```python
from build123d import *

# Parameters (mm, degrees)
SKETCH1_R           = 6.35
BOSS_EXTRUDE1_DEPTH = 22.86
SKETCH2_R           = 3.048
CUT_EXTRUDE1_DEPTH  = 8.636
SKETCH3_R           = 3.2385
CUT_EXTRUDE2_DEPTH  = 10.16


with BuildPart() as part:
    # Sketch1 → Boss-Extrude1 (new body)
    with BuildSketch(Plane(origin=(0, 0, 0), x_dir=(1, 0, 0), z_dir=(0, 1, 0))):
        Circle(SKETCH1_R)
    extrude(amount=BOSS_EXTRUDE1_DEPTH)

    # Sketch2 → Cut-Extrude1 (cut)
    with BuildSketch(Plane.XZ):
        Circle(SKETCH2_R)
    extrude(amount=-CUT_EXTRUDE1_DEPTH, mode=Mode.SUBTRACT)

    # Sketch3 → Cut-Extrude2 (cut)
    with BuildSketch(Plane(origin=(0, 22.86, 0), x_dir=(1, 0, 0), z_dir=(0, 1, 0))):
        Circle(SKETCH3_R)
    extrude(amount=-CUT_EXTRUDE2_DEPTH, mode=Mode.SUBTRACT)


solid = part.part
```
Design review of the part built by this model. Coordinates are the model's own, in mm. A direction names the side the tool comes from. Coordinates: 2 decimals unless noted, no trailing zeros. Order: outer loops, then holes, each group sorted by start corner. A loop starts at its lowest first (then second) coordinate and runs counter-clockwise, first axis right, second up. Notation, with made-up numbers: M 3,73 L 13,73 A29 cw 13,106 Z; hole C 71.25,23.5 d6. An arc over 180 degrees is marked long. Answer as a JSON object with one key per item and string values. Group by question number.
1) Add section A-A, the plane x = 0. Write out the cut boundary in (y, z).
2) Add section B-B, the plane z = 0. Write out the cut boundary in (x, y), then the cut area to 3 significant figures.
3) Wall thickness on L1, parallel to X at y = 19.5, z = 0; L2, parallel to Z at x = 0, y = 3.25: over which ranges is each line inside the solid? List them lowest first.
4) Add section C-C, the plane y = 7.5. Write out the cut boundary in (x, z), then the cut area to 3 significant figures.
5) Add section D-D, the plane y = 17. Write out the cut boundary in (x, z), then the cut area to 3 significant figures.
6) For pin 1 (4 mm diameter, centred on x = 0.5, y = 19.5, fed in from -Z); pin 2 (1.9 mm diameter, centred on x = 0, z = -1.5, fed in from +Y); pin 3 (3 mm diameter, centred on x = -3.5, y = 19, fed in from +Z); pin 4 (3 mm diameter, centred on y = 17.5, z = -3, fed in from -X), all flat-tipped, find the tip position at first contact; note any pin that passes through.
7) Tool access review of faces 1 (the flat face through (0, 12.7, 0)), 2 (the flat face through (0, 8.636, 0)), 3 (the flat face through (3, 0, -2)): name each direction out of +Z, -Z, +X, -X, +Y, -Y from which nothing blocks a thin tool from reaching the whole face with its end or side.
8) Mouldability with a two-part tool opening along X and no side actions: class faces 4 (the cylindrical face through (-1.38, 11.27, 6.2)), 5 (the cylindrical face through (-0.4, 4.26, 3.02)), 6 (the flat face through (-3, 22.86, -2)) as pulls with the +X half, pulls with the -X half, needs draft (parallel to the pull), parting line crosses it, or undercut.
Computed values:
{
 "1": {"outline": "M 0,-6.35 L 22.86,-6.35 L 22.86,-3.24 L 12.7,-3.24 L 12.7,3.24 L 22.86,3.24 L 22.86,6.35 L 0,6.35 L 0,3.05 L 8.64,3.05 L 8.64,-3.05 L 0,-3.05 Z"},
 "2": {"outline": "M -6.35,0 L -3.05,0 L -3.05,8.64 L 3.05,8.64 L 3.05,0 L 6.35,0 L 6.35,22.86 L 3.24,22.86 L 3.24,12.7 L -3.24,12.7 L -3.24,22.86 L -6.35,22.86 Z", "area": "172 mm^2"},
 "3": {"L1": "x = -6.35 to -3.24, 3.24 to 6.35", "L2": "z = -6.35 to -3.05, 3.05 to 6.35"},
 "4": {"outline": "C 0,0 d12.7; hole C 0,0 d6.1", "area": "97.5 mm^2"},
 "5": {"outline": "C 0,0 d12.7; hole C 0,0 d6.48", "area": "93.7 mm^2"},
 "6": {"pin 1": "stops at z = -6.35", "pin 2": "stops at y = 12.7", "pin 3": "stops at z = 6.03", "pin 4": "stops at x = -6.17"},
 "7": {"face 1": "+Y", "face 2": "-Y", "face 3": "+Z, -Z, +X, -X, -Y"},
 "8": {"face 4": "parting line crosses it", "face 5": "undercut", "face 6": "needs draft"}
}
